Check sheet for the modelled part. Datum: model origin and axes. Units: mm. Round coordinates to 2 decimals unless told otherwise and drop trailing zeros. Order: outer loops, then holes, each group sorted by start corner. A loop starts at its lowest first (then second) coordinate and runs counter-clockwise, first axis right, second up. Notation, with made-up numbers: M 48,13.5 L 97,13.5 A27 ccw 97,46.5 Z; hole C 70,-15 d7. An arc over 180 degrees is marked long. One line per item, written item: value. Start each with the question number.
(1) Release check for a two-part mould opening along Y. For faces 1 (the face through (6.084, -9.984, 3.251)), 2 (the face through (5.92, -1.29, -8.54)), 3 (the face through (6.084, 9.984, -3.251)) record: released by +Y, released by -Y, zero draft, split by the parting line, or undercut.
(2) Cross-section at A-A, the plane y = 0. Enter the section's corners in (x, z).
(3) Thickness scan on L1, parallel to Y at x = 0.25, z = 3.25; L2, parallel to Y at x = 1, z = 8.25; L3, parallel to X at y = 3.25, z = 0. Record the ranges inside material, lowest first.
(4) Cross-section at D-D, the plane x = -8.25. Enter the section's corners in (y, z), and give its area (3 significant figures).
(5) Depth check by flat-ended pin: pin 1 Ø3.5 at (x, z) = (-8.5, 0) entering from -Y; pin 2 Ø10 at (x, y) = (4, -3.5) entering from -Z; pin 3 Ø1.5 at (x, y) = (-7.5, 3.5) entering from +Z; pin 4 Ø4 at (x, z) = (-5, -7.5) entering from -Y. Enter the tip coordinate at first touch or a pass-through.
(6) Cross-section at B-B, the plane z = 0. Enter the section's corners in (x, y).
(7) Cross-section at C-C, the plane y = 5.25. Enter the section's corners in (x, z), and give its area (3 significant figures).
from build123d import *

# Parameters (mm, degrees)
BASPROSKE_W         = 12
BASPROSKE_H         = 10.5
TOOTHCUT_DEPTH      = 13
TEETHCUTS_COUNT     = 10
TEETHCUTS_ANGLE     = 324
BORSKE_R            = 2.5
BORE_DEPTH          = 50.0000508
SKETCH2_R           = 6
SKETCH2_R_2         = 2.75
BOSS_EXTRUDE1_DEPTH = 10
CUT_EXTRUDE1_DEPTH  = 10


with BuildPart() as part:
    # BasProSke → Base-Revolve (revolve)
    with BuildSketch(Plane(origin=(0, 0, 0), x_dir=(1, 0, 0), z_dir=(0, 1, 0))):
        with Locations((6, 5.25)):
            Rectangle(BASPROSKE_W, BASPROSKE_H)
    revolve(axis=Axis((-10, 0, 0), (1, 0, 0)))

    # TooCutSke → ToothCut (cut, through all)
    with BuildSketch(Plane(origin=(0, 0, 0), x_dir=(0, 0, -1), z_dir=(1, 0, 0))):
        with BuildLine():
            ThreePointArc((1.173901537, 6.455636098), (0, 6.5615), (-1.173901537, 6.455636098))
            ThreePointArc((-1.173901537, 6.455636098), (-1.430021039, 8.560346018), (-2.854248526, 10.131007379))
            ThreePointArc((-2.854248526, 10.131007379), (0, 10.5254), (2.854248526, 10.131007379))
            ThreePointArc((2.854248526, 10.131007379), (1.430021039, 8.560346018), (1.173901537, 6.455636098))
        make_face()
    toothcut = extrude(amount=TOOTHCUT_DEPTH, mode=Mode.SUBTRACT)

    # TeethCuts: ToothCut ×10 about axis
    teethcuts_axis = Axis((-10, 0, 0), (1, 0, 0))
    for i in range(1, TEETHCUTS_COUNT):
        add(toothcut.rotate(teethcuts_axis, i * TEETHCUTS_ANGLE / (TEETHCUTS_COUNT - 1)), mode=Mode.SUBTRACT)

    # BorSke → Bore (cut, symmetric)
    with BuildSketch(Plane(origin=(0, 0, 0), x_dir=(0, 0, -1), z_dir=(1, 0, 0))):
        Circle(BORSKE_R)
    extrude(amount=BORE_DEPTH, both=True, mode=Mode.SUBTRACT)

    # Sketch2 → Boss-Extrude1 (add)
    with BuildSketch(Plane.ZY):
        Circle(SKETCH2_R)
        Circle(SKETCH2_R_2, mode=Mode.SUBTRACT)
        with BuildLine():
            ThreePointArc((1.58113883, 2.25), (0.829156198, 2.62202212), (0, 2.75))
            Line((0, 2.75), (0, 2.5))
            ThreePointArc((0, 2.5), (0.559016994, 2.436698586), (1.089724736, 2.25))
            Line((1.089724736, 2.25), (1.58113883, 2.25))
        make_face()
        with BuildLine():
            Line((0, 2.5), (0, 2.75))
            ThreePointArc((0, 2.75), (-0.829156198, 2.62202212), (-1.58113883, 2.25))
            Line((-1.58113883, 2.25), (-1.089724736, 2.25))
            ThreePointArc((-1.089724736, 2.25), (-0.559016994, 2.436698586), (0, 2.5))
        make_face()
        with BuildLine():
            ThreePointArc((1.089724736, 2.25), (0.559016994, 2.436698586), (0, 2.5))
            Line((0, 2.5), (0, 2.25))
            Line((0, 2.25), (1.089724736, 2.25))
        make_face()
        with BuildLine():
            Line((0, 2.25), (0, 2.5))
            ThreePointArc((0, 2.5), (-0.559016994, 2.436698586), (-1.089724736, 2.25))
            Line((-1.089724736, 2.25), (0, 2.25))
        make_face()
    extrude(amount=BOSS_EXTRUDE1_DEPTH)

    # Sketch4 → Cut-Extrude1 (cut)
    with BuildSketch(Plane(origin=(0, 0, 0), x_dir=(1, 0, 0), z_dir=(0, 1, 0))):
        with BuildLine():
            ThreePointArc((-3.25, 0), (-5, 1.75), (-6.75, 0))
            Line((-6.75, 0), (-3.25, 0))
        make_face()
        with BuildLine():
            Line((-3.25, 0), (-6.75, 0))
            ThreePointArc((-6.75, 0), (-5, -1.75), (-3.25, 0))
        make_face()
    extrude(amount=CUT_EXTRUDE1_DEPTH, mode=Mode.SUBTRACT)


solid = part.part
Values found:
1. face 1: released by -Y
1. face 2: undercut
1. face 3: released by +Y
2. outline: M -10,-6 L 0,-6 L 0,-10.5 L 12,-10.5 L 12,-2.5 L 0,-2.5 L 0,-2.75 L -10,-2.75 Z; M -10,2.75 L 0,2.75 L 0,2.5 L 12,2.5 L 12,10.5 L 0,10.5 L 0,6 L -10,6 Z
3. L1: -9.98 to -6.37, -5.7 to 5.7, 6.37 to 9.98
3. L2: -6.5 to -4.65, -1.31 to 1.31, 4.65 to 6.5
3. L3: -10 to -6.75, -3.25 to 12
4. outline: C 0,0 d12; hole M 2.25,-1.58 L 2.25,1.58 A2.75 ccw long Z
4. area: 90.4 mm^2
5. pin 1: y = -6
5. pin 2: z = -10.5
5. pin 3: z = 5.33
5. pin 4: y = -2.4
6. outline: M -10,-6 L 0,-6 L 0,-6.56 L 12,-6.56 L 12,-2.5 L 0,-2.5 L 0,-2.75 L -10,-2.75 Z; M -10,2.25 L -6.75,2.25 L -6.75,6 L -10,6 Z; M -3.25,2.25 L 0,2.25 L 0,2.5 L 12,2.5 L 12,6.56 L 0,6.56 L 0,6 L -3.25,6 Z
7. outline: M -10,-2.9 L 0,-2.9 L 0,-3.94 L 12,-3.94 L 12,3.94 L 0,3.94 L 0,2.9 L -10,2.9 Z; M 0,-8.57 L 12,-8.57 L 12,-5.2 L 0,-5.2 Z; M 0,5.2 L 12,5.2 L 12,8.57 L 0,8.57 Z; hole C -5,0 d3.5
7. area: 224 mm^2
